from build123d import *

# Parameters (mm, degrees)
F0_W     = 234.95
F0_H     = 15.875
F1_DEPTH = 60.325
F2_W     = 6.35
F2_H     = 7.9375
F2_W_2   = 3
F3_DEPTH = 234.951
F5_DEPTH = 60.326


with BuildPart() as f1:
    # F0 (on Right) → F1 (new body)
    with BuildSketch(Plane.YZ):
        Rectangle(F0_W, F0_H)
    extrude(amount=F1_DEPTH)

    # F2 (on face) → F3 (cut, through all)
    with BuildSketch(Plane.XZ.offset(117.475)):
        with Locations((3.175, 3.96875)):
            Rectangle(F2_W, F2_H)
        with Locations((52.3, 3.96875)):
            Rectangle(F2_W_2, F2_H)
    extrude(amount=-F3_DEPTH, mode=Mode.SUBTRACT)

    # F4 (on face) → F5 (cut, through all)
    with BuildSketch(Plane.YZ.offset(60.325)):
        Polygon((-117.475, 7.9375), (-117.475, -7.9375), (-101.6, 7.9375), align=None)
        Polygon((101.6, 7.9375), (117.475, -7.9375), (117.475, 7.9375), align=None)
    extrude(amount=-F5_DEPTH, mode=Mode.SUBTRACT)


solid = f1.part
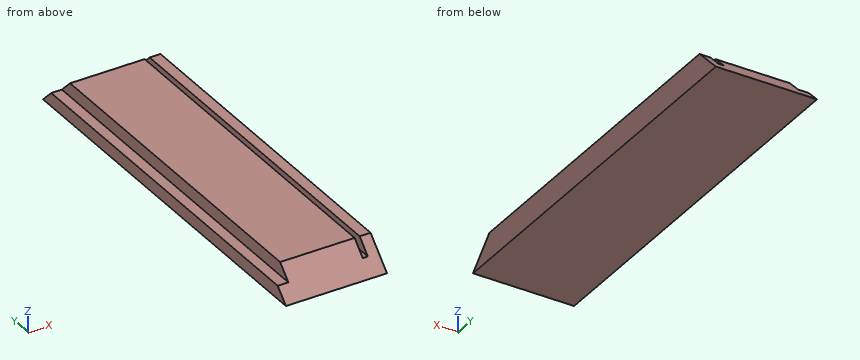
Build history of the part. All positions in model axes, mm. Coordinates: 2 decimals unless noted, no trailing zeros. Order: outer loops, then holes, each group sorted by start corner. A loop starts at its lowest first (then second) coordinate and runs counter-clockwise, first axis right, second up. Notation, with made-up numbers: (-14, -35.75) - (30, -35.75) arc R18 cw to (30, -14.75) - close; hole circle Ø8 at (13.25, 5). An arc over 180 degrees is marked (long way). Write each question's results on one line, items separated by ' | '. Start each with the question number.
Item 1: Band-saw the part on C-C on x = 36. Write the cut outline in (y, z) (1 decimal), and give its area (3 significant figures).
Item 2: Flat gauge pins, fed straight in: pin 1 (4 mm diameter, centred on y = -53.5, z = -4.5, fed in from -X); pin 2 (3 mm diameter, centred on x = 2.5, y = -20.5, fed in from +Z); pin 3 (5 mm diameter, centred on x = 51.5, z = -4.5, fed in from +Y); pin 4 (4 mm diameter, centred on y = -27.5, z = 4.5, fed in from -X). Where does each tip first touch, or does it go through?
Item 3: Wall check: probe 1 along X at (y, z) = (-10, 6.25) (3 decimals); probe 2 along Z at (x, y) = (13, -106.5); probe 3 along Y at (x, z) = (48.5, 0.25). Give the ranges that are in metal, low to high. Write a range as [from, to].
Numbers:
1) outline: (-117.5, -7.9) - (117.5, -7.9) - (101.6, 7.9) - (-101.6, 7.9) - close | area: 3,480 mm^2
2) pin 1: x = 0 | pin 2: z = 0 | pin 3: y = 116.54 | pin 4: x = 6.35
3) probe 1: [6.35, 50.8], [53.8, 60.325] | probe 2: [-7.94, 3.04] | probe 3: [-109.29, 109.29]
